Autodesk Inventor part; units mm, degrees
ref_plane "Work Plane1" through (17.9605, 0, 43.3605) normal (0.7071068, 0, 0.7071068) x (0.7071068, 0, -0.7071068)
ref_plane "Work Plane2" through (0, 0, 0) normal (0, 0, 1) x (1, 0, 0)
ref_plane "YZ Plane" through (0, 0, 0) normal (1, 0, 0) x (0, 1, 0)
sketch "Sketch1" plane through (0, 0, 0) normal (0, 1, 0) x (-1, 0, 0)
  line L0 (0, 0) -> (0, 25.4)
  line L1 (0, 25.4) -> (-17.9605, 43.3605)
  line L2 (-17.9605, 43.3605) -> (-30.0839, 31.2372) construction
  line L3 (-30.0839, 31.2372) -> (-12.1233, 13.2767) construction
  line L4 (0, 25.4) -> (-12.1233, 13.2767) construction
  line L5 (0, 25.4) -> (-17.145, 25.4) construction
  line L6 (-17.145, 25.4) -> (-17.145, 0) construction
  line L7 (0, 0) -> (-17.145, 0) construction
  line L8 (-17.145, 18.2983) -> (0, 25.4) construction
  line L9 (-17.145, 18.2983) -> (0, 18.2983) construction
  line L10 (-17.145, 18.2983) -> (-5.0217, 30.4217) construction
  line L11 (-17.9605, 43.3605) -> (-11.4831, 49.8379)
  line L12 (-11.4831, 49.8379) -> (-2.1972, 39.9528)
  line L13 (-2.1972, 39.9528) -> (0.8567, 43.0067)
  line L14 (0.8567, 43.0067) -> (9.2317, 34.6317)
  line L15 (0, 25.4) -> (9.2317, 34.6317)
  line L16 (-2.1972, 39.9528) -> (-8.375, 33.775) construction
  line L17 (0, 0) -> (9.1604, 0)
  line L18 (9.1604, 0) -> (8.7368, 13.556)
  line L19 (8.7368, 13.556) -> (13.0556, 13.556)
  line L20 (13.0556, 13.556) -> (13.0556, 25.4)
  line L21 (0, 25.4) -> (13.0556, 25.4)
  line L22 (8.7368, 13.556) -> (0, 13.556) construction
  dimension "d0" = 25.4
  dimension "d1" = 25.4
  dimension "d2" = 135
  dimension "d3" = 34.29
  dimension "d4" = 34.29
  dimension "d5" = 18.3208
  dimension "d6" = 26.1112
  dimension "d7" = 13.556
  dimension "d8" = 1.79
  dimension "d9" = 18.3208
  dimension "d10" = 26.1112
  dimension "d11" = 13.556
  dimension "d12" = 1.79
ref_plane "Work Plane1" through (17.9605, 0, 43.3605) normal (0.7071068, 0, 0.7071068) x (0.7071068, 0, -0.7071068)
ref_plane "Work Plane2" through (0, 0, 0) normal (0, 0, 1) x (1, 0, 0)
sketch "Sketch2" plane through (17.9605, 0, 43.3605) normal (0.7071068, 0, 0.7071068) x (0.7071068, 0, -0.7071068)
  circle A0 centre (0, 0) radius 17.145
  line L0 (0, 0) -> (17.145, 0)
  circle A1 centre (0, 0) radius 19.05
  dimension "d15" = 34.29
  dimension "d18" = 38.1
extrude "Extrude1" add sketch "Sketch2" against normal blind 25.4 contours A0
extrude "Extrude2" add sketch "Sketch2" against normal blind 19.812
sketch "Sketch3" plane through (0, 0, 0) normal (0, 0, 1) x (1, 0, 0)
  line L0 (0, 0) -> (17.145, 0)
  circle A0 centre (0, 0) radius 17.145
  circle A1 centre (0, 0) radius 19.05
  dimension "d22" = 34.29
  dimension "d25" = 38.1
extrude "Extrude3" add sketch "Sketch3" along normal blind 25.4 contours A0
extrude "Extrude4" add sketch "Sketch3" along normal blind 19.812
revolve "Revolve1" cut sketch "Sketch1" angle 360 about axis through (0, 0, 25.4) along (0.7071068, 0, 0.7071068) contours L1 L11 L12 L13 L14 L15
revolve "Revolve2" cut sketch "Sketch1" angle 360 about axis through (0, 0, 0) along (0, 0, 1) contours L0 L21 L20 L19 L18 L17
sketch "Sketch4" plane through (0, 0, 25.4) normal (0, 0, 1) x (1, 0, 0)
  arc A0 (0, 13.0556) -> (0, -13.0556) centre (0, 0) ccw
  line L0 (0, 17.145) -> (0, 13.0556)
  arc A1 (0, 17.145) -> (0, -17.145) centre (0, 0) ccw
  line L1 (0, -13.0556) -> (0, -17.145)
  arc A2 (0, 17.145) -> (0, -17.145) centre (0, 0) ccw
  arc A3 (0, 13.0556) -> (0, -13.0556) centre (0, 0) ccw
  line L2 (0, 13.0556) -> (0, -13.0556) construction
  line L3 (0, -13.0556) -> (0, -17.145)
  line L4 (0, 13.0556) -> (0, 17.145)
  dimension "d29" = 17.145
  dimension "d30" = 13.0556
revolve "Revolve3" add sketch "Sketch4" angle 45 about axis through (0, -13.0556, 25.4) along (0, 1, 0)
thread "Filetage1"
thread "Filetage2"
equation "\"d0\" = C1"
equation "\"d1\" = C1"
equation "\"d3\" = 0.9 * H"
equation "\"d4\" = 0.9 * H"
equation "\"d5\" = MD"
equation "\"d6\" = 0.9 * H - 2 * G"
equation "\"d7\" = L2"
equation "\"d9\" = MD"
equation "\"d10\" = 0.9 * H - 2 * G"
equation "\"d11\" = L2"
equation "\"d15\" = 0.9 * H"
equation "\"d18\" = H"
equation "\"d16\" = C1"
equation "\"d19\" = 0.78 * C1"
equation "\"d22\" = 0.9 * H"
equation "\"d25\" = H"
equation "\"d23\" = C1"
equation "\"d26\" = 0.78 * C1"
equation "\"d29\" = 0.45 * H"
equation "\"d30\" = 0.45 * H - G"
equation "\"C1\" = 25.4"
equation "\"H\" = 38.1"
equation "\"G\" = 4.0894"
equation "\"L2\" = 13.55598"
equation "\"MD\" = 18.32077"
equation "\"A\" = 33.274"
equation "\"Size_Designation\" = 0.5"
properties part number "ASME B16.11 Coude 45 deg taraudé - Catégorie 3000 1/2" material "Steel"
Part model, mm, in its own coordinate system. A direction names the side the tool comes from. Give positions to 0.01 mm unless a question says otherwise; leave off trailing zeros. Write each loop counter-clockwise with the first axis right and the second up, starting at its lowest first coordinate (ties: lowest second). Pieces come first, ordered by that corner, then holes. Notation, with made-up numbers: (-18, 1.5) -> (38, 1.5) arc R36 cw to (38, 38.5) -> close; hole circle Ø5 at (55, -18.5). An arc over 180 degrees is marked (long way). Put each result on its own line as item: value. Start each with the question number.
Item 1: Cut at A-A (y = 0). List the corners of the cut face in (x, z) (3 decimals), then the cut area to 3 significant figures.
Item 2: Pin check, flat tips, straight feed: pin 1 Ø13 at (x, y) = (-3, 4) entering from +Z; pin 2 Ø5 at (x, z) = (-7, 21) entering from +Y; pin 3 Ø3 at (x, z) = (15.5, 15) entering from +Y. Stop position of each tip, or through.
Item 3: Cut at C-C (y = 15.5). List the corners of the cut face in (x, z).
Item 4: Pull direction X, two halves, no side cores. Call faces 3 (the face through (7.197, -2.689, 44.672)), 4 (the face through (8, 5, 0)), 5 (the face through (23.76, 4.5, 37.56)): pulls with the +X half, pulls with the -X half, needs draft (parallel to the pull), parting line crosses it, or undercut.
Item 5: Cut at B-B (z = 9). List the corners of the cut face in (x, y), then the cut area to 3 significant figures.
Item 6: Wall check: L1, parallel to Y at x = 0, z = 19.5; L2, parallel to Y at x = 0, z = 23 (3 decimals); L3, parallel to Z at x = -11, y = -5. Give the ranges that are in metal, low to high. Write a range as [from, to].
Item 7: Which spindle directions (+Z, -Z, +X, -X, +Y, -Y) get a long thin tool onto all of the face, cutting with end or side? Do faces 1 (the face through (-8.3, 0.1, 41.6)), 2 (the face through (1.94, -8.74, 6.68)). Say none if no direction does.
Answer list:
1. outline: (-19.05, 0) -> (-9.16, 0) -> (-8.737, 13.556) -> (-13.056, 13.556) -> (-13.056, 25.4) arc R13.056 cw to (-9.232, 34.632) -> (-0.857, 43.007) -> (2.197, 39.953) -> (11.483, 49.838) -> (4.49, 56.831) -> (-9.519, 42.822) -> (-8.172, 41.475) -> (-12.123, 37.523) arc R17.145 ccw to (-17.145, 25.4) -> (-17.145, 19.812) -> (-19.05, 19.812) -> close; (8.737, 13.556) -> (9.16, 0) -> (19.05, 0) -> (19.05, 17.509) -> (31.431, 29.89) -> (24.438, 36.883) -> (14.553, 27.597) -> (17.607, 24.543) -> (13.056, 19.992) -> (13.056, 13.556) -> close
1. area: 779 mm2
2. pin 1: stops at z = 55.44
2. pin 2: stops at y = 18.44
2. pin 3: stops at y = 12.92
3. outline: (-11.07, 0) -> (11.07, 0) -> (11.07, 19.81) -> (7.33, 19.81) -> (7.33, 22.36) -> (9.13, 24.17) -> (11.78, 21.52) -> (25.79, 35.53) -> (10.13, 51.19) -> (-3.88, 37.18) -> (-1.23, 34.53) -> (-5.18, 30.58) arc R7.33 ccw to (-7.33, 25.4) -> (-7.33, 19.81) -> (-11.07, 19.81) -> close
4. face 3: undercut
4. face 4: needs draft
4. face 5: pulls with the +X half
5. outline: circle Ø38.1 at (0, 0); hole circle Ø17.76 at (0, 0)
5. area: 892 mm2
6. L1: y = [-19.05, -13.06], [13.06, 19.05]
6. L2: y = [-17.145, -13.056], [13.056, 17.145]
6. L3: z = [0, 13.56], [30.34, 37.59]
7. face 1: none
7. face 2: -Z
